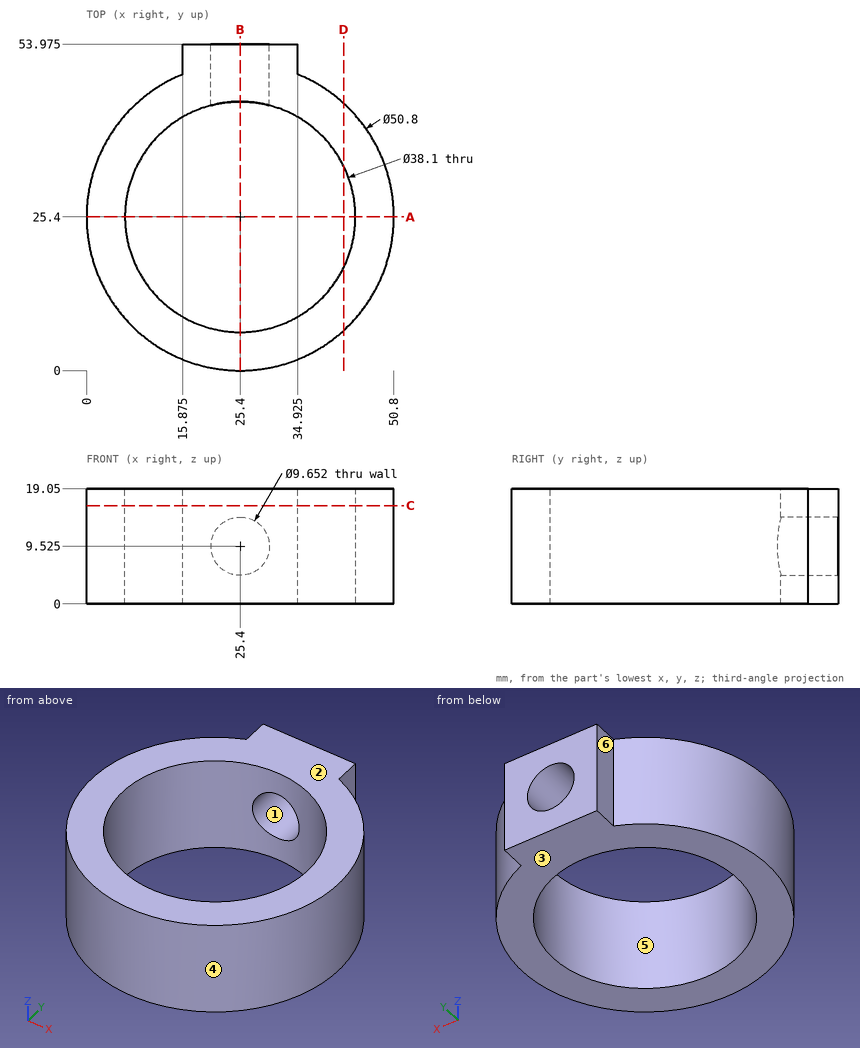
Design review of the part shown in the three views and the two pictorial views. Dimensions are in mm from the part's minimum x, y and z. A direction names the side the tool comes from. Coordinates: 2 decimals unless noted, no trailing zeros. Loops run counter-clockwise (first coordinate to the right, second up) from the corner with the lowest first, then second, coordinate; pieces in that order, holes last. Notation, with made-up numbers: (10, 72.5) -> (60, 72.5) arc R25 cw to (60, 85.5) -> close; hole circle Ø6 at (46, -40). An arc over 180 degrees is marked (long way). Answer as CSV lines item,"result".
Item 1: Machinability: for the marked faces 5 and 6, which of the approach directions +Z, -Z, +X, -X, +Y, -Y give a long, thin tool a straight path to every point of the face, cutting with its end or side? Answer none if there is none.
Results below:
face 5,"+Z, -Z"
face 6,"+Z, -Z, -X, +Y"
Item 2: Take a section at C-C, the plane z = 16.25. State the section outline as (x, y) points (3 decimals).
Results below:
outline,"(15.875, 48.946) arc R25.4 ccw (long way) to (34.925, 48.946) -> (34.925, 53.975) -> (15.875, 53.975) -> close; hole circle Ø38.1 at (25.4, 25.4)"
Item 3: Take a section at D-D, the plane x = 42.5. State the section outline as (y, z) points, and give its area (3 significant figures).
Results below:
outline,"(6.62, 0) -> (17, 0) -> (17, 19.05) -> (6.62, 19.05) -> close; (33.8, 0) -> (44.18, 0) -> (44.18, 19.05) -> (33.8, 19.05) -> close"
area,"396 mm2"
Item 4: Take a section at A-A, the plane y = 25.4. State the section outline as (x, z) points, and give its area (3 significant figures).
Results below:
outline,"(0, 0) -> (6.35, 0) -> (6.35, 19.05) -> (0, 19.05) -> close; (44.45, 0) -> (50.8, 0) -> (50.8, 19.05) -> (44.45, 19.05) -> close"
area,"242 mm2"
Item 5: Insertion check: pin 1 (2 mm diameter, centred on x = 40.5, z = 9.5, fed in from -Y); pin 2 (10 mm diameter, centred on x = 6.5, z = 11, fed in from -Y); pin 3 (1.5 mm diameter, centred on y = 50.5, z = 5, fed in from +X) (3 decimals). Each pin has a flat end and moves straight along its axis. Give the tip position at first contact, or say it passes through.
Results below:
pin 1,"stops at y = 4.27"
pin 2,"stops at y = 4.14"
pin 3,"stops at x = 34.925"
Item 6: Draft analysis for pull direction Z (two halves, no side actions). For the marked faces 1, 2, 3 and 4, state which applies: +Z half, -Z half, draft (parallel to the pull), parting line (faces both ways), or undercut.
Results below:
face 1,"undercut"
face 2,"+Z half"
face 3,"-Z half"
face 4,"draft"
Item 7: For L1, parallel to Y at x = 38.5, z = 10.5; L2, parallel to X at y = 49, z = 3.25 (3 decimals); L3, parallel to Y at x = 11, z = 1.5, list the stretches that pass through material, from the lowest coordinate up.
Results below:
L1,"y = 3.64 to 11.57, 39.23 to 47.16"
L2,"x = 15.875 to 34.925"
L3,"y = 4.48 to 12.93, 37.87 to 46.32"
Item 8: Take a section at B-B, the plane x = 25.4. State the section outline as (y, z) points (3 decimals).
Results below:
outline,"(0, 0) -> (6.35, 0) -> (6.35, 19.05) -> (0, 19.05) -> close; (44.45, 0) -> (53.975, 0) -> (53.975, 4.699) -> (44.45, 4.699) -> close; (44.45, 14.351) -> (53.975, 14.351) -> (53.975, 19.05) -> (44.45, 19.05) -> close"
